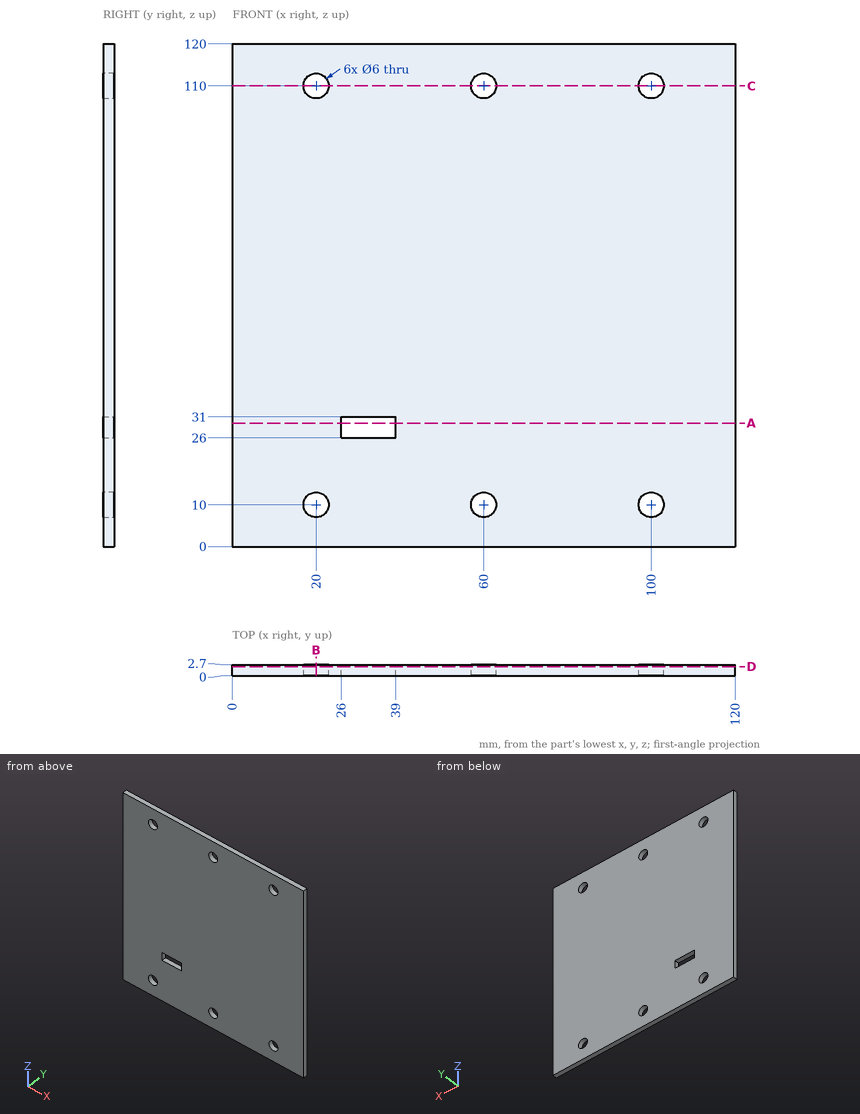
The drawing under review shows one solid part. Ordinate dimensions are in mm from its lowest x, y, z. Round coordinates to 2 decimals unless told otherwise and drop trailing zeros. Write each loop counter-clockwise with the first axis right and the second up, starting at its lowest first coordinate (ties: lowest second). Pieces come first, ordered by that corner, then holes. Notation, with made-up numbers: (7.5, 70.5) -> (22.5, 70.5) arc R21 cw to (22.5, 77.5) -> close; hole circle Ø1 at (43.25, 52). An arc over 180 degrees is marked (long way). One line per question, with ' | ' between items.
(1) Insertion check: P1, Ø2, axis at x = 91, z = 104.5, coming from the -Y side. The pin has a flat end and moves straight along its axis. Give the tip position at first contact, or say it passes through.
Result sheet:
P1: y = 0
(2) Take a section at C-C, the plane z = 110. State the section outline as (x, y) points, and give its area (3 significant figures).
Result sheet:
outline: (0, 0) -> (17, 0) -> (17, 2.7) -> (0, 2.7) -> close; (23, 0) -> (57, 0) -> (57, 2.7) -> (23, 2.7) -> close; (63, 0) -> (97, 0) -> (97, 2.7) -> (63, 2.7) -> close; (103, 0) -> (120, 0) -> (120, 2.7) -> (103, 2.7) -> close | area: 275 mm2
(3) Take a section at D-D, the plane y = 2.25. State the section outline as (x, z) points, and give its area (3 significant figures).
Result sheet:
outline: (0, 0) -> (120, 0) -> (120, 120) -> (0, 120) -> close; hole circle Ø6 at (20, 10); hole circle Ø6 at (20, 110); hole (26, 26) -> (39, 26) -> (39, 31) -> (26, 31) -> close; hole circle Ø6 at (60, 10); hole circle Ø6 at (60, 110); hole circle Ø6 at (100, 10); hole circle Ø6 at (100, 110) | area: 14,200 mm2
(4) Take a section at B-B, the plane x = 20. State the section outline as (y, z) points, and give its area (3 significant figures).
Result sheet:
outline: (0, 0) -> (2.7, 0) -> (2.7, 7) -> (0, 7) -> close; (0, 13) -> (2.7, 13) -> (2.7, 107) -> (0, 107) -> close; (0, 113) -> (2.7, 113) -> (2.7, 120) -> (0, 120) -> close | area: 292 mm2
(5) Wall thickness on line 1 (X direction, y = 1.95, z = 10); line 2 (Z direction, x = 19, y = 1.85); line 3 (Z direction, x = 36, y = 1.6): over which ranges is each line inside the solid? List them lowest first. Write a range as [from, to].
Result sheet:
line 1: [0, 17], [23, 57], [63, 97], [103, 120] | line 2: [0, 7.17], [12.83, 107.17], [112.83, 120] | line 3: [0, 26], [31, 120]
(6) Take a section at A-A, the plane z = 29.5. State the section outline as (x, y) points, and give its area (3 significant figures).
Result sheet:
outline: (0, 0) -> (26, 0) -> (26, 2.7) -> (0, 2.7) -> close; (39, 0) -> (120, 0) -> (120, 2.7) -> (39, 2.7) -> close | area: 289 mm2
